```python
from build123d import *

# Parameters (mm, degrees)
SKETCH1_R           = 4.7
SKETCH1_R_2         = 3.2
BOSS_EXTRUDE1_DEPTH = 10
SKETCH2_R           = 7
BOSS_EXTRUDE2_DEPTH = 6
SKETCH3_R           = 6
CUT_EXTRUDE1_DEPTH  = 4
SKETCH4_R           = 3.2
CUT_EXTRUDE2_DEPTH  = 15.071247279
CHAMFER2_SIZE       = 1.5
CHAMFER4_SIZE       = 3
CHAMFER5_SIZE       = 1


with BuildPart() as part:
    # Sketch1 → Boss-Extrude1 (new body)
    with BuildSketch(Plane(origin=(0, 0, 0), x_dir=(1, 0, 0), z_dir=(0, 1, 0))):
        with Locations(Location((0, 0, 0), (0, 0, 270))):
            Circle(SKETCH1_R)
        with Locations(Location((0, 0, 0), (0, 0, 270))):
            Circle(SKETCH1_R_2, mode=Mode.SUBTRACT)
    extrude(amount=BOSS_EXTRUDE1_DEPTH)

    # Sketch2 → Boss-Extrude2 (add)
    with BuildSketch(Plane(origin=(0, 0, 0), x_dir=(1, 0, 0), z_dir=(0, 1, 0))):
        with Locations(Location((0, 0, 0), (0, 0, 270))):
            Circle(SKETCH2_R)
    extrude(amount=-BOSS_EXTRUDE2_DEPTH)

    # Sketch3 → Cut-Extrude1 (cut)
    with BuildSketch(Plane.XZ.offset(6)):
        with Locations(Location((0, 0, 0), (0, 0, 270))):
            Circle(SKETCH3_R)
    extrude(amount=-CUT_EXTRUDE1_DEPTH, mode=Mode.SUBTRACT)

    # Sketch4 → Cut-Extrude2 (cut, through all)
    with BuildSketch(Plane(origin=(0, 0, 0), x_dir=(1, 0, 0), z_dir=(0, 1, 0))):
        with Locations(Location((0, 0, 0), (0, 0, 270))):
            Circle(SKETCH4_R)
    extrude(amount=-CUT_EXTRUDE2_DEPTH, mode=Mode.SUBTRACT)

    # Chamfer2
    # the kernel refuses this chamfer: 1.5 mm, written as the material it takes off along each edge
    with BuildSketch(Plane(origin=(0, -6, 0), x_dir=(0, 0, 1), z_dir=(-1, 0, 0))) as chamfer2_piece_1:
        Polygon((7, CHAMFER2_SIZE), (7 - CHAMFER2_SIZE, 0), (7, 0), align=None)
    revolve(axis=Axis((0, -6, 0), (0, 1, 0)), mode=Mode.SUBTRACT)

    # Chamfer4
    # the kernel refuses this chamfer: 3 mm, written as the material it adds along each edge
    with BuildSketch(Plane(origin=(0, 0, 0), x_dir=(0, 0, 1), z_dir=(-1, 0, 0))) as chamfer4_piece_1_section:
        Polygon((4.7 + CHAMFER4_SIZE, 0), (4.7, CHAMFER4_SIZE), (4.7, 0), align=None)
    chamfer4_piece_1 = revolve(axis=Axis((0, 0, 0), (0, 1, 0)), mode=Mode.PRIVATE)
    chamfer4_piece_1 = chamfer4_piece_1 & Plane(origin=(0, 1.853894362, 0), x_dir=(0, 0, 1), z_dir=(0, 1, 0)) * Cylinder(7, 31, mode=Mode.PRIVATE)
    add(chamfer4_piece_1)

    # Chamfer5
    chamfer5_edges = [part.edges().sort_by_distance(p)[0] for p in [
        (0, -2, -3.2),
    ]]
    chamfer(chamfer5_edges, length=CHAMFER5_SIZE)


solid = part.part
```
Read the model definition and answer for the solid it produces. Units are mm, in the model's axes. A direction names the side the tool comes from. Round coordinates to 2 decimals unless told otherwise and drop trailing zeros. Write each loop counter-clockwise with the first axis right and the second up, starting at its lowest first coordinate (ties: lowest second). Pieces come first, ordered by that corner, then holes. Notation, with made-up numbers: (17, 68) -> (21, 68) arc R14 cw to (21, 93) -> close; hole circle Ø11 at (-7, -35.75). An arc over 180 degrees is marked (long way). Answer in a Markdown table with one row per item. Add a question column.
1) Which of the six approach directions +Z, -Z, +X, -X, +Y, -Y give full straight-line access (tool end or side, diameter ignored) to faces 4 (the face through (4.77, 2.89, -0.63)), 5 (the face through (-4, -2, -3))?
2) Determine the mould class of faces 1 (the face through (-3, 10, 2)), 2 (the face through (1.802, -3.774, -5.723)), 3 (the face through (1.412, 6.451, 4.483)) for opening direction Z: pulls with the +Z half, pulls with the -Z half, needs draft (parallel to the pull), parting line crosses it, or undercut.
3) Find section C-C, the plane y = 1.5. Determine the outline of the cut face in (x, z), and give its area (3 significant figures).
4) Consider line 1 (X direction, y = -0.7, z = 0); line 2 (X direction, y = 3.75, z = 0); line 3 (Z direction, x = 0.25, y = 8.5). Determine where each line is inside the solid, lowest interval first.
5) Find section D-D, the plane y = 4. Determine the outline of the cut face in (x, z).
6) Find section B-B, the plane z = 0. Determine the outline of the cut face in (x, y).
7) Given P1, Ø5, axis at y = 7, z = -4.5, coming from the +X side; P2, Ø8, axis at x = 5.5, y = 0.5, coming from the +Z side; P3, Ø5, axis at y = 5.5, z = 2.5, coming from the -X side; P4, Ø5, axis at x = 0, z = 0, coming from the -Y side, each flat-ended and moving along its own axis, determine where each tip first touches the part or whether it passes through.
8) Find section A-A, the plane x = 0. Determine the outline of the cut face in (y, z).
Findings below:
| question | item | result |
|---|---|---|
| 1 | face 4 | +Y |
| 1 | face 5 | -Y |
| 2 | face 1 | needs draft |
| 2 | face 2 | undercut |
| 2 | face 3 | parting line crosses it |
| 3 | outline | circle Ø12.4 at (0, 0); hole circle Ø6.4 at (0, 0) |
| 3 | area | 88.6 mm² |
| 4 | line 1 | -7 to -3.2, 3.2 to 7 |
| 4 | line 2 | -4.7 to -3.2, 3.2 to 4.7 |
| 4 | line 3 | -4.69 to -3.19, 3.19 to 4.69 |
| 5 | outline | circle Ø9.4 at (0, 0); hole circle Ø6.4 at (0, 0) |
| 6 | outline | (-7, -4.5) -> (-6, -5.5) -> (-6, -2) -> (-4.2, -2) -> (-3.2, -1) -> (-3.2, 10) -> (-4.7, 10) -> (-4.7, 3) -> (-7, 0.7) -> close; (3.2, -1) -> (4.2, -2) -> (6, -2) -> (6, -5.5) -> (7, -4.5) -> (7, 0.7) -> (4.7, 3) -> (4.7, 10) -> (3.2, 10) -> close |
| 7 | P1 | x = 4.25 |
| 7 | P2 | z = 6.84 |
| 7 | P3 | x = -4.7 |
| 7 | P4 | through |
| 8 | outline | (-5.5, -6) -> (-4.5, -7) -> (0.7, -7) -> (3, -4.7) -> (10, -4.7) -> (10, -3.2) -> (-1, -3.2) -> (-2, -4.2) -> (-2, -6) -> close; (-5.5, 6) -> (-2, 6) -> (-2, 4.2) -> (-1, 3.2) -> (10, 3.2) -> (10, 4.7) -> (3, 4.7) -> (0.7, 7) -> (-4.5, 7) -> close |
